Read the model definition and answer for the solid it produces. Units are mm, in the model's axes. Coordinates: 2 decimals unless noted, no trailing zeros. Order: outer loops, then holes, each group sorted by start corner. A loop starts at its lowest first (then second) coordinate and runs counter-clockwise, first axis right, second up. Notation, with made-up numbers: (50.5, 31.25) -> (59.5, 31.25) arc R11 cw to (59.5, 45.25) -> close; hole circle Ø9 at (6.5, -32.5). An arc over 180 degrees is marked (long way). Answer as a JSON object with one key per item and string values. Group by question number.
1) Given pin 1 (1 mm diameter, centred on x = 1.5, z = -119, fed in from -Y); pin 2 (2 mm diameter, centred on y = -135, z = 188, fed in from -X), each flat-ended and moving along its own axis, determine where each tip first touches the part or whether it passes through.
2) Consider L1, parallel to Y at x = 4.05, z = -265; L2, parallel to Y at x = 2.8, z = 187; L3, parallel to Z at x = 2, y = 518. Determine where each line is inside the solid, lowest interval first.
3) Section B-B on z = 242.5 is taken. Determine the outline of the cut face in (x, y).
4) Section A-A on x = 3.15 is taken. Determine the outline of the cut face in (y, z).
Autodesk Inventor part; units mm, degrees
ref_plane "YZ Plane" through (0, 0, 0) normal (1, 0, 0) x (0, 1, 0)
ref_plane "XZ Plane" through (0, 0, 0) normal (0, 1, 0) x (-1, 0, 0)
ref_plane "XY Plane" through (0, 0, 0) normal (0, 0, 1) x (1, 0, 0)
sketch "Boceto1" plane through (0, 0, 0) normal (1, 0, 0) x (0, 1, 0)
  line L0 (-522.3171, 332.4506) -> (-488.1102, -337.5494)
  line L1 (561.6295, -332.4506) -> (527.4226, 337.5494)
  line L2 (-472.3821, 385) -> (477.4876, 385)
  line L3 (-438.1752, -385) -> (511.6946, -385)
  arc A0 (-472.3821, 385) -> (-522.3171, 332.4506) centre (-472.3821, 335) ccw
  arc A1 (-488.1102, -337.5494) -> (-438.1752, -385) centre (-438.1752, -335) ccw
  arc A2 (511.6946, -385) -> (561.6295, -332.4506) centre (511.6946, -335) ccw
  arc A3 (527.4226, 337.5494) -> (477.4876, 385) centre (477.4876, 335) ccw
  point P0 (0, 0)
  point P1 (-525, 385)
  point P2 (525, 385)
  point P3 (-485.6876, -385)
  point P4 (564.3124, -385)
  dimension "d17" = 1050
  dimension "d19" = 1050
  dimension "d20" = 770
  dimension "d21" = 385
  dimension "d22" = 525
  dimension "d23" = 50
  dimension "d24" = 50
extrude "Extrusión1" add sketch "Boceto1" along normal blind 5
properties part number "Ventanas"
Worked answers:
{
 "1": {"pin 1": "stops at y = -499.29", "pin 2": "stops at x = 0"},
 "2": {"L1": "y = -491.81 to 558.19", "L2": "y = -514.89 to 535.11", "L3": "z = -384.6 to 364.3"},
 "3": {"outline": "(0, -517.72) -> (5, -517.72) -> (5, 532.28) -> (0, 532.28) -> close"},
 "4": {"outline": "(-522.32, 332.45) -> (-488.11, -337.55) arc R50 ccw to (-438.18, -385) -> (511.69, -385) arc R50 ccw to (561.63, -332.45) -> (527.42, 337.55) arc R50 ccw to (477.49, 385) -> (-472.38, 385) arc R50 ccw to start"}
}
